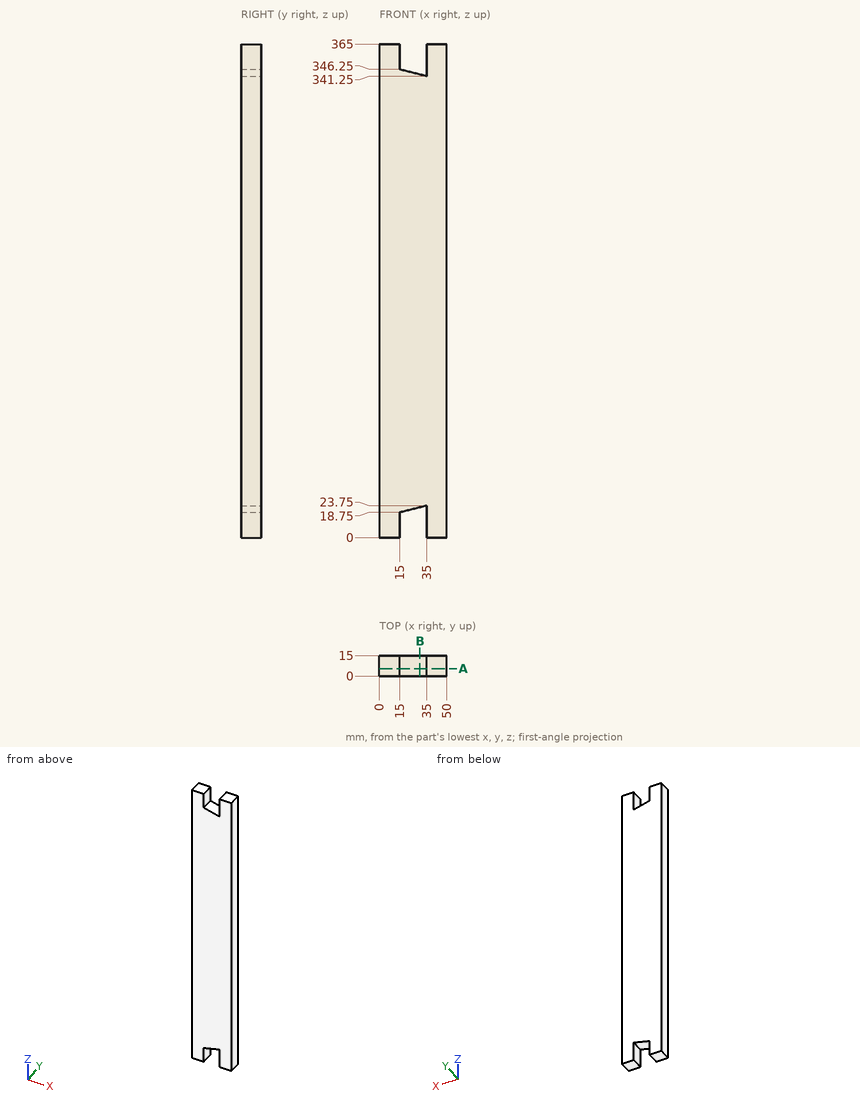
Print and shaded views of the part. All mm, measured from the part's lowest x, y and z. Round coordinates to 2 decimals unless told otherwise and drop trailing zeros. Write each loop counter-clockwise with the first axis right and the second up, starting at its lowest first coordinate (ties: lowest second). Pieces come first, ordered by that corner, then holes. Notation, with made-up numbers: (22.25, 16.5) - (65.25, 16.5) arc R17 cw to (65.25, 49.5) - close; hole circle Ø9 at (-4.5, 9). An arc over 180 degrees is marked (long way). Write each question's results on one line, items separated by ' | '. Start each with the question number.
Item 1: Wall check: L1, parallel to Z at x = 33, y = 10; L2, parallel to Z at x = 29.5, y = 10.25 (3 decimals). Give the ranges that are in metal, low to high. Write a range as [from, to].
Item 2: Drop a flat-ended pin along its axis: P1, Ø12, axis at x = 10, z = 171.5, coming from the -Y side. Give the stop position or say it passes through.
Item 3: Saw through at A-A (y = 5.5). Write the cut outline in (x, z).
Item 4: Saw through at B-B (x = 30). Write the cut outline in (y, z), and give its area (3 significant figures).
Results are:
1) L1: z = [23.25, 341.75] | L2: z = [22.375, 342.625]
2) P1: stops at y = 0
3) outline: (0, 0) - (15, 0) - (15, 18.75) - (35, 23.75) - (35, 0) - (50, 0) - (50, 365) - (35, 365) - (35, 341.25) - (15, 346.25) - (15, 365) - (0, 365) - close
4) outline: (0, 22.5) - (15, 22.5) - (15, 342.5) - (0, 342.5) - close | area: 4,800 mm²
